Model file for the job. Use its own axes, mm. Face numbers are marked on the shaded views. A direction names the side the tool comes from. Coordinates: 2 decimals unless noted, no trailing zeros. Write each loop counter-clockwise with the first axis right and the second up, starting at its lowest first coordinate (ties: lowest second). Pieces come first, ordered by that corner, then holes. Notation, with made-up numbers: (70.5, 28) - (122.5, 28) arc R7 ccw to (122.5, 35) - close; hole circle Ø8 at (1, -21.75). An arc over 180 degrees is marked (long way). Put each result on its own line as item: value. Start each with the question number.
1. Drill centre lines: L1, parallel to X at y = 2.25, z = 38; L2, parallel to Z at x = 16.5, y = 3.5; L3, parallel to X at y = 9, z = 11.5. Where is each one in solid material? Low to high. Write a range as from..to.
2. Pull direction Z, two halves, no side cores. Call the marked faces 1, 2, 3 and 4: released by +Z, released by -Z, zero draft, split by the parting line, or undercut.
3. Saw through at B-B, the plane y = 6.5. Give the number of separate pieces and of enclosed holes in the cut face, plus the area to 3 significant figures.
4. Saw through at D-D, the plane z = -26. Write the cut outline in (x, y), plus the area to 3 significant figures.
5. Saw through at A-A, the plane x = -1.5. Write the cut outline in (y, z).
6. Which spindle directions (+Z, -Z, +X, -X, +Y, -Y) get a long thin tool onto all of the face, cutting with end or side? Do the marked faces 5, 6 and 7. Say none if no direction does.
7. Drop flat-ended pins along their axis: P1, Ø2.5, axis at x = 24.5, z = -37, coming from the +Y side; P2, Ø16.5, axis at x = -9.5, y = 6, coming from the -Z side; P3, Ø10, axis at y = 24, z = -5.5, coming from the +X side. Give the stop position or say it passes through.
8. Saw through at C-C, the plane z = 2. Write the cut outline in (x, y).
```python
from build123d import *

# Parameters (mm, degrees)
SKETCH1_R             = 2.5
SKETCH1_R_2           = 1.25
BOSS_EXTRUDE1_DEPTH   = 10
BOSS_EXTRUDE1_2_DEPTH = 10
BOSS_EXTRUDE1_3_DEPTH = 10
BOSS_EXTRUDE1_4_DEPTH = 10
SKETCH2_W             = 68
SKETCH2_H             = 98
BOSS_EXTRUDE2_DEPTH   = 3
SKETCH3_W             = 68
SKETCH3_H             = 98
SKETCH3_W_2           = 64
SKETCH3_H_2           = 94
BOSS_EXTRUDE3_DEPTH   = 30
SKETCH4_R             = 6.2
CUT_EXTRUDE1_DEPTH    = 25
CUT_EXTRUDE2_DEPTH    = 5
SKETCH7_R             = 3.5
BOSS_EXTRUDE5_DEPTH   = 33
SKETCH8_R             = 1
CUT_EXTRUDE3_DEPTH    = 7
CUT_EXTRUDE6_DEPTH    = 3.3
CUT_EXTRUDE7_DEPTH    = 10


with BuildPart() as part:
    # Sketch1 → Boss-Extrude1 (new body)
    with BuildSketch(Plane(origin=(0, 0, 0), x_dir=(1, 0, 0), z_dir=(0, 1, 0))):
        with Locations(Location((24.328009845, -38, 0), (0, 0, 270))):
            Circle(SKETCH1_R)
        with Locations(Location((24.328009845, -38, 0), (0, 0, 270))):
            Circle(SKETCH1_R_2, mode=Mode.SUBTRACT)
    extrude(amount=BOSS_EXTRUDE1_DEPTH)



with BuildPart() as body_2:
    # Sketch1 → Boss-Extrude1 2 (new body)
    with BuildSketch(Plane(origin=(0, 0, 0), x_dir=(1, 0, 0), z_dir=(0, 1, 0))):
        with Locations(Location((24.328009845, 38, 0), (0, 0, 270))):
            Circle(SKETCH1_R)
        with Locations(Location((24.328009845, 38, 0), (0, 0, 270))):
            Circle(SKETCH1_R_2, mode=Mode.SUBTRACT)
    extrude(amount=BOSS_EXTRUDE1_2_DEPTH)


with BuildPart() as body_3:
    # Sketch1 → Boss-Extrude1 3 (new body)
    with BuildSketch(Plane(origin=(0, 0, 0), x_dir=(1, 0, 0), z_dir=(0, 1, 0))):
        with Locations(Location((-22.671990155, 38, 0), (0, 0, 270))):
            Circle(SKETCH1_R)
        with Locations(Location((-22.671990155, 38, 0), (0, 0, 270))):
            Circle(SKETCH1_R_2, mode=Mode.SUBTRACT)
    extrude(amount=BOSS_EXTRUDE1_3_DEPTH)


with BuildPart() as body_4:
    # Sketch1 → Boss-Extrude1 4 (new body)
    with BuildSketch(Plane(origin=(0, 0, 0), x_dir=(1, 0, 0), z_dir=(0, 1, 0))):
        with Locations(Location((-22.671990155, -38, 0), (0, 0, 270))):
            Circle(SKETCH1_R)
        with Locations(Location((-22.671990155, -38, 0), (0, 0, 270))):
            Circle(SKETCH1_R_2, mode=Mode.SUBTRACT)
    extrude(amount=BOSS_EXTRUDE1_4_DEPTH)


with BuildPart() as part_1:
    add(part.part)

    add(body_2.part)  # Boss-Extrude2 merges body 2

    add(body_3.part)  # Boss-Extrude2 merges body 3

    add(body_4.part)  # Boss-Extrude2 merges body 4
    # Sketch2 → Boss-Extrude2 (add)
    with BuildSketch(Plane(origin=(0, 0, 0), x_dir=(1, 0, 0), z_dir=(0, 1, 0))):
        with Locations((0.828009845, 0)):
            Rectangle(SKETCH2_W, SKETCH2_H)
    extrude(amount=-BOSS_EXTRUDE2_DEPTH)

    # Sketch3 → Boss-Extrude3 (add)
    with BuildSketch(Plane(origin=(0, 0, 0), x_dir=(1, 0, 0), z_dir=(0, 1, 0))):
        with Locations((0.828009845, 0)):
            Rectangle(SKETCH3_W, SKETCH3_H)
        with Locations((0.828009845, 0)):
            Rectangle(SKETCH3_W_2, SKETCH3_H_2, mode=Mode.SUBTRACT)
    extrude(amount=BOSS_EXTRUDE3_DEPTH)

    # Sketch4 → Cut-Extrude1 (cut)
    with BuildSketch(Plane.XY.offset(49)):
        with Locations((23.028009845, 21.2)):
            Circle(SKETCH4_R)
    extrude(amount=-CUT_EXTRUDE1_DEPTH, mode=Mode.SUBTRACT)

    # Sketch5 → Cut-Extrude2 (cut)
    with BuildSketch(Plane.ZY.offset(33.171990155)):
        with BuildLine():
            Line((42.5, 19.5), (31.5, 19.5))
            ThreePointArc((31.5, 19.5), (28.318019485, 18.181980515), (27, 15))
            Line((27, 15), (37, 15))
            Line((37, 15), (47, 15))
            ThreePointArc((47, 15), (45.681980515, 18.181980515), (42.5, 19.5))
        make_face()
        with BuildLine():
            Line((37, 15), (27, 15))
            ThreePointArc((27, 15), (28.318019485, 11.818019485), (31.5, 10.5))
            Line((31.5, 10.5), (37, 10.5))
            Line((37, 10.5), (37, 15))
        make_face()
        with BuildLine():
            ThreePointArc((42.5, 10.5), (45.681980515, 11.818019485), (47, 15))
            Line((47, 15), (37, 15))
            Line((37, 15), (37, 10.5))
            Line((37, 10.5), (42.5, 10.5))
        make_face()
    extrude(amount=-CUT_EXTRUDE2_DEPTH, mode=Mode.SUBTRACT)

    # Sketch7 → Boss-Extrude5 (add)
    with BuildSketch(Plane(origin=(0, 30, 0), x_dir=(1, 0, 0), z_dir=(0, 1, 0))):
        with Locations((32.828009845, -47)):
            Circle(SKETCH7_R)
        with Locations((32.828009845, 47)):
            Circle(SKETCH7_R)
        with Locations((-31.171990155, 47)):
            Circle(SKETCH7_R)
        with Locations((-31.171990155, -47)):
            Circle(SKETCH7_R)
    extrude(amount=-BOSS_EXTRUDE5_DEPTH)

    # Sketch8 → Cut-Extrude3 (cut)
    with BuildSketch(Plane(origin=(0, 30, 0), x_dir=(1, 0, 0), z_dir=(0, 1, 0))):
        with Locations(Location((-31.171990155, -47, 0), (0, 0, 270))):
            Circle(SKETCH8_R)
        with Locations(Location((32.828009845, -47, 0), (0, 0, 270))):
            Circle(SKETCH8_R)
        with Locations(Location((32.828009845, 47, 0), (0, 0, 270))):
            Circle(SKETCH8_R)
        with Locations(Location((-31.171990155, 47, 0), (0, 0, 270))):
            Circle(SKETCH8_R)
    extrude(amount=-CUT_EXTRUDE3_DEPTH, mode=Mode.SUBTRACT)

    # Sketch12 → Cut-Extrude6 (cut)
    with BuildSketch(Plane(origin=(0, 0, -49), x_dir=(-1, 0, 0), z_dir=(0, 0, -1))):
        with BuildLine():
            Line((-20.828009845, 25), (19.171990155, 25))
            ThreePointArc((19.171990155, 25), (26.671990155, 17.5), (19.171990155, 10))
            Line((19.171990155, 10), (-20.828009845, 10))
            ThreePointArc((-20.828009845, 10), (-28.328009845, 17.5), (-20.828009845, 25))
        make_face()
    extrude(amount=-CUT_EXTRUDE6_DEPTH, mode=Mode.SUBTRACT)

    # Sketch14 → Cut-Extrude7 (cut)
    with BuildSketch(Plane(origin=(34.828009845, 0, 0), x_dir=(0, 0, -1), z_dir=(1, 0, 0))):
        with BuildLine():
            Line((8.633857568, 25), (35.621579786, 25))
            ThreePointArc((35.621579786, 25), (43.121579786, 17.5), (35.621579786, 10))
            Line((35.621579786, 10), (8.633857568, 10))
            ThreePointArc((8.633857568, 10), (1.133857568, 17.5), (8.633857568, 25))
        make_face()
    extrude(amount=-CUT_EXTRUDE7_DEPTH, mode=Mode.SUBTRACT)


solid = part_1.part
```
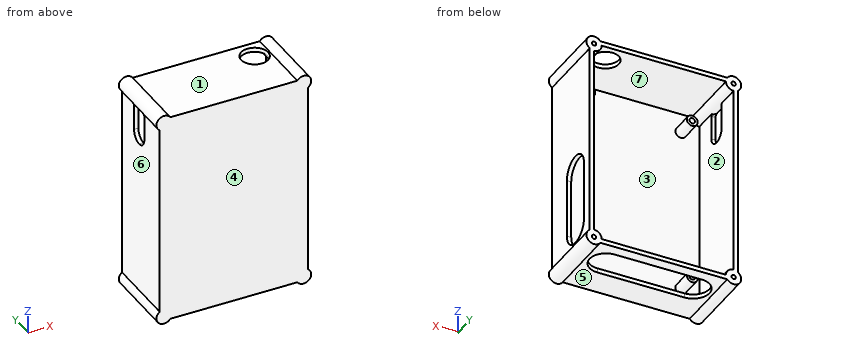
Final values:
1. L1: x = -33.17..-31.17, -25.17..-23.92, -21.42..-20.17, 21.83..23.08, 25.58..26.83, 32.83..34.83
1. L2: z = -49..-47, 47..49
1. L3: x = -33.17..-31.17, 32.83..34.83
2. face 1: released by +Z
2. face 2: undercut
2. face 3: undercut
2. face 4: zero draft
3. separate pieces: 5
3. enclosed holes: 5
3. area: 792 mm²
4. outline: (-33.17, -3) - (34.83, -3) - (34.83, 10) - (32.83, 10) - (32.83, 0) - (-31.17, 0) - (-31.17, 30) - (-33.17, 30) - close; (32.83, 25) - (34.83, 25) - (34.83, 30) - (32.83, 30) - close
4. area: 294 mm²
5. outline: (-3, -49) - (10, -49) - (10, -47) - (0, -47) - (0, 47) - (30, 47) - (30, 49) - (-3, 49) - close; (25, -49) - (30, -49) - (30, -47) - (25, -47) - close
6. face 5: -Z, +Y, -Y
6. face 6: -X, +Y, -Y
6. face 7: +Y
7. P1: stops at y = 10
7. P2: stops at z = -49
7. P3: stops at x = 34.83
8. outline: (-33.17, -3) - (34.83, -3) - (34.83, 30) - (32.83, 30) - (32.83, 0) - (-31.17, 0) - (-31.17, 30) - (-33.17, 30) - close
